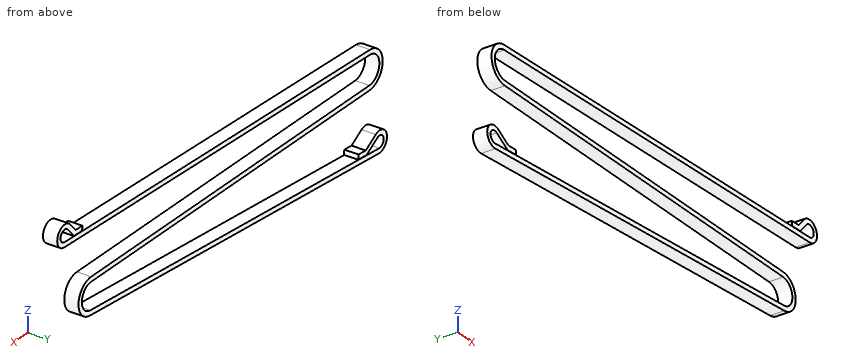
from build123d import *

# Parameters (mm, degrees)
EXTRUDE_THIN1_DEPTH = 3


with BuildPart() as part:
    # Sketch2 → Extrude-Thin1 (new, symmetric)
    with BuildSketch(Plane(origin=(0, 19.326776695, 0), x_dir=(1, 0, 0), z_dir=(0, 1, 0))):
        with BuildLine():
            Line((83.328079119, -22.116037785), (88.322896843, -22.343624921))
            Line((88.322896843, -22.343624921), (91.997250324, -26.627587507))
            ThreePointArc((91.997250324, -26.627587507), (96.141958225, -26.095715612), (94.008663166, -22.502591138))
            Line((94.008663166, -22.502591138), (-90.364139419, -14.101708358))
            ThreePointArc((-90.364139419, -14.101708358), (-97.997143033, -5.896216694), (-89.936648421, 1.889749157))
            Line((-89.936648421, 1.889749157), (77.956049842, 0.560174022))
            ThreePointArc((77.956049842, 0.560174022), (83.543259885, 5.836559245), (78.502463441, 11.6372082))
            Line((78.502463441, 11.6372082), (-95.878795519, 27.489733424))
            ThreePointArc((-95.878795519, 27.489733424), (-98.545913109, 24.45909356), (-94.848135548, 22.838990066))
            Line((-94.848135548, 22.838990066), (-88.221929105, 26.693256199))
            Line((-88.221929105, 26.693256199), (-83.242462258, 26.240586433))
            Line((-83.242462258, 26.240586433), (-83.423530164, 24.248799694))
            Line((-83.423530164, 24.248799694), (-87.767727276, 24.643718819))
            Line((-87.767727276, 24.643718819), (-93.842539664, 21.110182118))
            ThreePointArc((-93.842539664, 21.110182118), (-100.498539275, 24.026368407), (-95.697727612, 29.481520162))
            Line((-95.697727612, 29.481520162), (78.683531348, 13.628994939))
            ThreePointArc((78.683531348, 13.628994939), (85.540831015, 5.738022037), (77.940211947, -1.439763267))
            Line((77.940211947, -1.439763267), (-89.952486316, -0.110188132))
            ThreePointArc((-89.952486316, -0.110188132), (-95.997857275, -5.949662521), (-90.273104564, -12.103781269))
            Line((-90.273104564, -12.103781269), (94.099698021, -20.504664048))
            ThreePointArc((94.099698021, -20.504664048), (97.939629126, -26.972288102), (90.479154905, -27.929657512))
            Line((90.479154905, -27.929657512), (87.367872452, -24.302184627))
            Line((87.367872452, -24.302184627), (83.237044264, -24.113964874))
            Line((83.237044264, -24.113964874), (83.328079119, -22.116037785))
        make_face()
    extrude(amount=EXTRUDE_THIN1_DEPTH, both=True)


solid = part.part
Could you check a few things on this model? Use its own coordinates, in mm. Give positions to 0.01 mm unless a question says otherwise; leave off trailing zeros. Loops run counter-clockwise (first coordinate to the right, second up) from the corner with the lowest first, then second, coordinate; pieces in that order, holes last. Notation, with made-up numbers: M 88,-25.5 L 105,-25.5 A7 cw 105,-20.5 Z; hole C 45,67 d8. An arc over 180 degrees is marked long. Answer as a JSON object with one key per item and string values.
Q1. Suppose I cut it at B-B, the plane x = -14. List the corners of the cut face in (y, z) for me, plus the area to 3 significant figures.
Values found:
{"outline": "M 16.33,-22.05 L 22.33,-22.05 L 22.33,-20.05 L 16.33,-20.05 Z; M 16.33,-1.29 L 22.33,-1.29 L 22.33,0.71 L 16.33,0.71 Z; M 16.33,15.58 L 22.33,15.58 L 22.33,17.58 L 16.33,17.58 Z", "area": "36.1 mm²"}
Q2. Suppose I cut it at A-A, the plane y = 21.35. List the corners of the cut face in (x, z) for me.
Values found:
{"outline": "M -95.88,-27.49 A2.5 cw long -94.85,-22.84 L -88.22,-26.69 L -83.24,-26.24 L -83.42,-24.25 L -87.77,-24.64 L -93.84,-21.11 A4.5 ccw long -95.7,-29.48 L 78.68,-13.63 A7.55 ccw 77.94,1.44 L -89.95,0.11 A6 cw -90.27,12.1 L 94.1,20.5 A4.5 ccw long 90.48,27.93 L 87.37,24.3 L 83.24,24.11 L 83.33,22.12 L 88.32,22.34 L 92,26.63 A2.5 cw long 94.01,22.5 L -90.36,14.1 A8 ccw -89.94,-1.89 L 77.96,-0.56 A5.55 cw 78.5,-11.64 Z"}
Q3. For P1, Ø6, axis at x = -34.5, z = 11, coming from the +Y side; P2, Ø6.5, axis at x = 93.89, z = 25, coming from the -Y side; P3, Ø2, axis at x = 61.5, y = 20, coming from the -Z side; P4, Ø1.5, axis at x = -30.5, y = 21.5, coming from the +Z side, each with a flat end and sliding along its axis, tell me the tip position at first contact or that it passes through.
Values found:
{"P1": "passes through", "P2": "stops at y = 16.33", "P3": "stops at z = -15.28", "P4": "stops at z = 16.86"}
Q4. Suppose I cut it at C-C, the plane z = -6.11. List the corners of the cut face in (x, y) for me.
Values found:
{"outline": "M 83.55,16.33 L 85.55,16.33 L 85.55,22.33 L 83.55,22.33 Z"}
Q5. If I drill on probe 1 along Z at (x, y) = (29, 19.15); probe 2 along Z at (x, y) = (3, 20.45); probe 3 along X at (y, z) = (20.8, 25), over which ranges is the centre line in solid material (lowest first)? Write a range as [from, to].
Values found:
{"probe 1": "z = [-18.15, -16.14], [-0.95, 1.05], [17.54, 19.54]", "probe 2": "z = [-20.51, -18.5], [-1.15, 0.85], [16.35, 18.36]", "probe 3": "x = [87.97, 90.6], [96.39, 98.39]"}
Q6. Suppose I cut it at D-D, the plane z = 7. List the corners of the cut face in (x, y) for me.
Values found:
{"outline": "M -97.95,16.33 L -95.93,16.33 L -95.93,22.33 L -97.95,22.33 Z"}
